The listing builds one solid part. Answer for the finished solid, in the listing's coordinates (mm). A direction names the side the tool comes from. Give positions to 0.01 mm unless a question says otherwise; leave off trailing zeros. Loops run counter-clockwise (first coordinate to the right, second up) from the corner with the lowest first, then second, coordinate; pieces in that order, holes last. Notation, with made-up numbers: M 35,-18 L 41,-18 A8 ccw 41,-11 Z; hole C 77,-28.75 d7. An arc over 180 degrees is marked long. Use one line per item in the form item = value. Start each with the question number.
1. The part is cut by section A-A (z = 2.5). Write down the section's boundary in (x, y).
2. For faces 1 (the face through (0, 0, 0)), 2 (the face through (2.29, 0.72, 2.56)), determine the directions among +Z, -Z, +X, -X, +Y, -Y from which every point of the face is accessible in a straight line to the end or side of a thin tool.
3. Straight lines are drawn through the part: line 1 (Y direction, x = 0.1, z = 3.5); line 2 (X direction, y = -1.4, z = 5.75); line 3 (Z direction, x = 1.6, y = 0.95). For each, find the intervals that lie inside material, in ascending order. Write a range as from..to.
from build123d import *

# Parameters (mm, degrees)
F0_R     = 2.4
F1_DEPTH = 10
F3_DEPTH = 4
F5_DEPTH = 2
F6_R     = 1.9999


# Not quite as in the source:
# - a fillet or chamfer is up to 0.001 mm smaller than in the source, because OpenCascade refuses the exact size
# - a feature names something its author has since deleted; it is built from what else it names


with BuildPart() as f1:
    # F0 (on Top) → F1 (new body)
    with BuildSketch(Plane.XY):
        Circle(F0_R)
    extrude(amount=F1_DEPTH)

    # F2 (on Front) → F3 (cut, symmetric)
    with BuildSketch(Plane.XZ):
        Polygon((-2.5, 10.5), (-2.5, 4.75), (2.5, 6.75), (2.5, 10.5), align=None)
    extrude(amount=F3_DEPTH, both=True, mode=Mode.SUBTRACT)

    # F4 (on face) → F5 (join)
    with BuildSketch(Plane(origin=(-1.9827586207, 0, 4.9568965517), x_dir=(0.9284766909, 0, 0.3713906764), z_dir=(-0.3713906764, 0, 0.9284766909))):
        with BuildLine():
            add(Edge.make_bspline(
                [(2.135496578, 2.4), (4.7203754965, 2.3999998246), (4.7203754965, 0)],
                knots=[7.8915744057, 7.8915744057, 7.8915744057, 9.4247779608, 9.4247779608, 9.4247779608], degree=2, weights=[0.8038475615, 0.6339746132, 1]))
            add(Edge.make_bspline(
                [(2.1354967017, -2.4), (1.4428802648, -2.4000000778), (0.8430568353, -2.0784609691), (-3.0342618258, 0), (0.8430568353, 2.0784609691), (1.4428802074, 2.400000047), (2.135496578, 2.4)],
                knots=[4.6747961621, 4.6747961621, 4.6747961621, 5.235987756, 5.235987756, 7.3303828584, 7.3303828584, 7.8915744057, 7.8915744057, 7.8915744057], degree=2, weights=[0.8038475512, 0.8660253757, 1, 0.5, 1, 0.8660253868, 0.8038475615]))
            add(Edge.make_bspline(
                [(4.7203754965, 0), (4.7203754965, -2.3999997097), (2.1354967017, -2.4)],
                knots=[3.1415926536, 3.1415926536, 3.1415926536, 4.6747961621, 4.6747961621, 4.6747961621], degree=2, weights=[1, 0.6339746243, 0.8038475512]))
        make_face()
    extrude(amount=F5_DEPTH)

    # F6 (radius 2 in the source; OpenCascade refuses exactly that, so slightly less here)
    f6_edges = [f1.edges().sort_by_distance(p)[0] for p in [
        (1.029171, -1.618698, 8.315734),
        (-3.142781, 0, 6.646953),
        (1.029171, 1.618698, 8.315734),
    ]]
    fillet(f6_edges, radius=F6_R)


solid = f1.part
Derived:
q1.outline = C 0,0 d4.8
q2.face_1 = -Z, +X, -X, +Y, -Y
q2.face_2 = -Z
q3.line_1 = -2.4..2.4
q3.line_2 = -2.05..1.95
q3.line_3 = 0..7.42
